Geometry: final body of the model. Coordinates: model frame, mm. Face numbers are marked on the shaded views. A direction names the side the tool comes from. Give positions to 0.01 mm unless a question says otherwise; leave off trailing zeros. Write each loop counter-clockwise with the first axis right and the second up, starting at its lowest first coordinate (ties: lowest second). Pieces come first, ordered by that corner, then holes.
Q1. Section D-D (z = 21.5). Return the cut outline in (x, y).
Q2. Line query: line 1 (Y direction, x = 11, z = 11.25); line 2 (Y direction, x = 21.25, z = 18). Output: solid intervals per line, ascending.
Q3. Section C-C (x = 19). Return the cut outline in (y, z), plus the area to 3 significant figures.
Q4. Section B-B (z = 9.25). Return the cut outline in (x, y), plus the area to 3 significant figures.
Q5. Pin query (flat end, axial travel): pin 1 Ø5 at (x, y) = (7, 13.5) entering from -Z; pin 2 Ø1 at (y, z) = (5.5, 4) entering from +X. Return the tip coordinate at first contact, or that it passes through.
Q6. Mould query, pull axis Z, two halves, no side actions, for the marked faces 1, 2 and 3. Classes: +Z half, -Z half, draft (parallel to the pull), parting line (faces both ways), or undercut.
Q7. Section A-A (y = 16.5). Return the cut outline in (x, z), plus the area to 3 significant figures.
Q8. Reachability of the marked faces 4 and 5 from +Z, -Z, +X, -X, +Y, -Y: full face, straight path, thin tool, end or side. Return the list, or none.
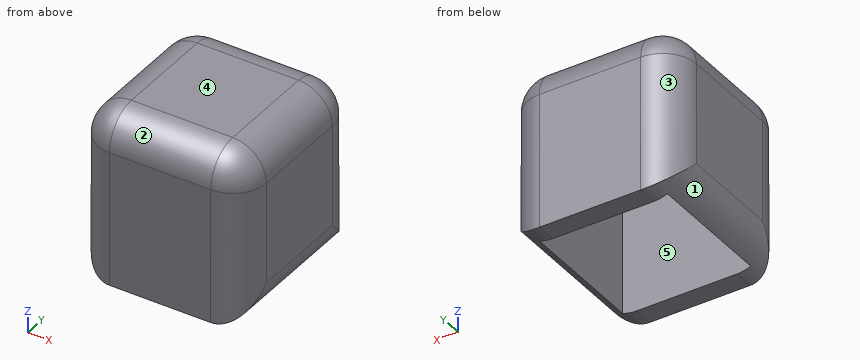
from build123d import *

# Parameters (mm, degrees)
F0_W         = 25
F0_H         = 25
F1_DEPTH     = 25
F2_T         = -3
F3_T1_DEPTH  = 32.5
F3_T3_DEPTH  = 50
F3_T5_DEPTH  = 15
F3_T7_DEPTH  = 15
F3_S11_W     = 5
F3_S11_H     = 5
F3_T12_DEPTH = 5
F3_S17_W     = 5
F3_S17_H     = 5
F3_T18_DEPTH = 5
F3_S23_W     = 5
F3_S23_H     = 5
F3_T24_DEPTH = 5
F3_S29_W     = 5
F3_S29_H     = 5
F3_T30_DEPTH = 5


# Not quite as in the source:
# - a fillet or chamfer that OpenCascade refuses, or shapes differently, is made with other operations: its cross-section is extruded or revolved along the edge and cut away or added


with BuildPart() as f1:
    # F0 (on Top) → F1 (new body)
    with BuildSketch(Plane.XY):
        with Locations((12.5, 12.5)):
            Rectangle(F0_W, F0_H)
    extrude(amount=F1_DEPTH)

    # F2
    f2_openings = [f1.faces().sort_by_distance(p)[0] for p in [
        (12.5, 12.5, 0),
    ]]
    offset(amount=F2_T, openings=f2_openings)

    # F3: fillet of radius 5 on 10 edges, made by hand

    # F3_s2 → F3_t1 (cut)
    with BuildSketch(Plane.XY.offset(-12.5)):
        with BuildLine():
            ThreePointArc((25, 20), (23.5355339059, 23.5355339059), (20, 25))
            Line((20, 25), (25, 25))
            Line((25, 25), (25, 20))
        make_face()
        with BuildLine():
            ThreePointArc((20, 0), (23.5355339059, 1.4644660941), (25, 5))
            Line((25, 5), (25, 0))
            Line((25, 0), (20, 0))
        make_face()
        with BuildLine():
            ThreePointArc((0, 20), (1.4644660941, 23.5355339059), (5, 25))
            Line((5, 25), (0, 25))
            Line((0, 25), (0, 20))
        make_face()
        with BuildLine():
            ThreePointArc((0, 5), (1.4644660941, 1.4644660941), (5, 0))
            Line((5, 0), (0, 0))
            Line((0, 0), (0, 5))
        make_face()
    extrude(amount=F3_T1_DEPTH, mode=Mode.SUBTRACT)

    # F3_s4 → F3_t3 (cut)
    with BuildSketch(Plane.XZ.offset(-37.5)):
        with BuildLine():
            ThreePointArc((25, 5), (23.5355339059, 1.4644660941), (20, 0))
            Line((20, 0), (25, 0))
            Line((25, 0), (25, 5))
        make_face()
        with BuildLine():
            ThreePointArc((0, 5), (1.4644660941, 1.4644660941), (5, 0))
            Line((5, 0), (0, 0))
            Line((0, 0), (0, 5))
        make_face()
    extrude(amount=F3_T3_DEPTH, mode=Mode.SUBTRACT)

    # F3_s6 → F3_t5 (cut)
    with BuildSketch(Plane.XZ.offset(-20)):
        with BuildLine():
            ThreePointArc((25, 20), (23.5355339059, 23.5355339059), (20, 25))
            Line((20, 25), (25, 25))
            Line((25, 25), (25, 20))
        make_face()
        with BuildLine():
            ThreePointArc((0, 20), (1.4644660941, 23.5355339059), (5, 25))
            Line((5, 25), (0, 25))
            Line((0, 25), (0, 20))
        make_face()
    extrude(amount=F3_T5_DEPTH, mode=Mode.SUBTRACT)

    # F3_s8 → F3_t7 (cut)
    with BuildSketch(Plane.YZ.offset(5)):
        with BuildLine():
            ThreePointArc((0, 20), (1.4644660941, 23.5355339059), (5, 25))
            Line((5, 25), (0, 25))
            Line((0, 25), (0, 20))
        make_face()
        with BuildLine():
            ThreePointArc((25, 20), (23.5355339059, 23.5355339059), (20, 25))
            Line((20, 25), (25, 25))
            Line((25, 25), (25, 20))
        make_face()
    extrude(amount=F3_T7_DEPTH, mode=Mode.SUBTRACT)


with BuildPart() as f3_tool10:
    # F3_s11 → F3_t12 (new body)
    with BuildSketch(Plane.YZ.offset(20)):
        with Locations((22.5, 22.5)):
            Rectangle(F3_S11_W, F3_S11_H)
    extrude(amount=F3_T12_DEPTH)

    # F3_s13 → F3_t14 (revolve, cut)
    with BuildSketch(Plane(origin=(20, 20, 20), x_dir=(0, -0.7071067812, -0.7071067812), z_dir=(0, -0.7071067812, 0.7071067812))):
        with BuildLine():
            ThreePointArc((0, -5), (5, 0), (0, 5))
            Line((0, 5), (0, -5))
        make_face()
    revolve(axis=Axis((20, 20, 20), (1, 0, 0)), mode=Mode.SUBTRACT)


with BuildPart() as f1_1:
    add(f1.part)

    # F3_t9: cut F3_tool10
    add(f3_tool10.part, mode=Mode.SUBTRACT)


with BuildPart() as f3_tool16:
    # F3_s17 → F3_t18 (new body)
    with BuildSketch(Plane.XZ.offset(-5)):
        with Locations((22.5, 22.5)):
            Rectangle(F3_S17_W, F3_S17_H)
    extrude(amount=F3_T18_DEPTH)

    # F3_s19 → F3_t20 (revolve, cut)
    with BuildSketch(Plane(origin=(20, 5, 20), x_dir=(-0.7071067812, 0, -0.7071067812), z_dir=(-0.7071067812, 0, 0.7071067812))):
        with BuildLine():
            ThreePointArc((0, -5), (5, 0), (0, 5))
            Line((0, 5), (0, -5))
        make_face()
    revolve(axis=Axis((20, 5, 20), (0, -1, 0)), mode=Mode.SUBTRACT)


with BuildPart() as f1_2:
    add(f1_1.part)

    # F3_t15: cut F3_tool16
    add(f3_tool16.part, mode=Mode.SUBTRACT)


with BuildPart() as f3_tool22:
    # F3_s23 → F3_t24 (new body)
    with BuildSketch(Plane.YZ.offset(5)):
        with Locations((22.5, 22.5)):
            Rectangle(F3_S23_W, F3_S23_H)
    extrude(amount=-F3_T24_DEPTH)

    # F3_s25 → F3_t26 (revolve, cut)
    with BuildSketch(Plane(origin=(5, 20, 20), x_dir=(0, -0.7071067812, -0.7071067812), z_dir=(0, 0.7071067812, -0.7071067812))):
        with BuildLine():
            ThreePointArc((0, -5), (5, 0), (0, 5))
            Line((0, 5), (0, -5))
        make_face()
    revolve(axis=Axis((5, 20, 20), (-1, 0, 0)), mode=Mode.SUBTRACT)


with BuildPart() as f1_3:
    add(f1_2.part)

    # F3_t21: cut F3_tool22
    add(f3_tool22.part, mode=Mode.SUBTRACT)


with BuildPart() as f3_tool28:
    # F3_s29 → F3_t30 (new body)
    with BuildSketch(Plane.YZ.offset(5)):
        with Locations((2.5, 22.5)):
            Rectangle(F3_S29_W, F3_S29_H)
    extrude(amount=-F3_T30_DEPTH)

    # F3_s31 → F3_t32 (revolve, cut)
    with BuildSketch(Plane(origin=(5, 5, 20), x_dir=(0, 0.7071067812, -0.7071067812), z_dir=(0, 0.7071067812, 0.7071067812))):
        with BuildLine():
            ThreePointArc((0, -5), (5, 0), (0, 5))
            Line((0, 5), (0, -5))
        make_face()
    revolve(axis=Axis((5, 5, 20), (-1, 0, 0)), mode=Mode.SUBTRACT)


with BuildPart() as f1_4:
    add(f1_3.part)

    # F3_t27: cut F3_tool28
    add(f3_tool28.part, mode=Mode.SUBTRACT)


solid = f1_4.part
Computed:
1. outline: (0.23, 5) arc R4.77 ccw to (5, 0.23) - (20, 0.23) arc R4.77 ccw to (24.77, 5) - (24.77, 20) arc R4.77 ccw to (20, 24.77) - (5, 24.77) arc R4.77 ccw to (0.23, 20) - close; hole (3, 3) - (22, 3) - (22, 22) - (3, 22) - close
2. line 1: y = 0 to 3, 22 to 25
2. line 2: y = 0.16 to 3, 22 to 24.84
3. outline: (0, 0) - (3, 0) - (3, 22) - (22, 22) - (22, 0) - (25, 0) - (25, 20) arc R5 ccw to (20, 25) - (5, 25) arc R5 ccw to (0, 20) - close
3. area: 196 mm2
4. outline: (0, 5) arc R5 ccw to (5, 0) - (20, 0) arc R5 ccw to (25, 5) - (25, 20) arc R5 ccw to (20, 25) - (5, 25) arc R5 ccw to (0, 20) - close; hole (3, 3) - (22, 3) - (22, 22) - (3, 22) - close
4. area: 243 mm2
5. pin 1: stops at z = 22
5. pin 2: stops at x = 24.97
6. face 1: -Z half
6. face 2: +Z half
6. face 3: draft
7. outline: (0, 5) arc R5 ccw to (3, 0.42) - (3, 22) - (22, 22) - (22, 0.42) arc R5 ccw to (25, 5) - (25, 20) arc R5 ccw to (20, 25) - (5, 25) arc R5 ccw to (0, 20) - close
7. area: 186 mm2
8. face 4: +Z, +X, -X, +Y, -Y
8. face 5: -Z
